The listing builds one solid part. Answer for the finished solid, in the listing's coordinates (mm). A direction names the side the tool comes from. Coordinates: 2 decimals unless noted, no trailing zeros. Order: outer loops, then holes, each group sorted by start corner. A loop starts at its lowest first (then second) coordinate and runs counter-clockwise, first axis right, second up.
```python
from build123d import *

# Parameters (mm, degrees)
SKETCH1_W           = 25.4
SKETCH1_H           = 50.8
SKETCH1_W_2         = 19.05
SKETCH1_H_2         = 44.45
BOSS_EXTRUDE1_DEPTH = 431.8
SKETCH2_R           = 2.54
CUT_EXTRUDE1_DEPTH  = 436.519276267
SKETCH3_R           = 2.54
CUT_EXTRUDE2_DEPTH  = 436.519276267


with BuildPart() as part:
    # Sketch1 → Boss-Extrude1 (new body)
    with BuildSketch(Plane.XY):
        with Locations((12.7, 25.4)):
            Rectangle(SKETCH1_W, SKETCH1_H)
        with Locations((12.7, 25.4)):
            Rectangle(SKETCH1_W_2, SKETCH1_H_2, mode=Mode.SUBTRACT)
    extrude(amount=BOSS_EXTRUDE1_DEPTH)

    # Sketch2 → Cut-Extrude1 (cut, through all)
    with BuildSketch(Plane(origin=(0, 50.8, 0), x_dir=(1, 0, 0), z_dir=(0, 1, 0))):
        with Locations(Location((12.7, -12.7, 0), (0, 0, 270))):
            Circle(SKETCH2_R)
        with Locations(Location((13.029725146, -25.4, 0), (0, 0, 270))):
            Circle(SKETCH2_R)
        with Locations(Location((13.029725146, -38.1, 0), (0, 0, 270))):
            Circle(SKETCH2_R)
        with Locations(Location((13.029725146, -406.4, 0), (0, 0, 270))):
            Circle(SKETCH2_R)
        with Locations(Location((13.029725146, -419.1, 0), (0, 0, 270))):
            Circle(SKETCH2_R)
        with Locations(Location((13.029725146, -393.7, 0), (0, 0, 270))):
            Circle(SKETCH2_R)
        with Locations(Location((13.029725146, -368.3, 0), (0, 0, 270))):
            Circle(SKETCH2_R)
        with Locations(Location((13.029725146, -317.5, 0), (0, 0, 270))):
            Circle(SKETCH2_R)
        with Locations(Location((13.029725146, -266.7, 0), (0, 0, 270))):
            Circle(SKETCH2_R)
        with Locations(Location((13.029725146, -215.9, 0), (0, 0, 270))):
            Circle(SKETCH2_R)
        with Locations(Location((13.029725146, -165.1, 0), (0, 0, 270))):
            Circle(SKETCH2_R)
        with Locations(Location((13.029725146, -114.3, 0), (0, 0, 270))):
            Circle(SKETCH2_R)
        with Locations(Location((13.029725146, -63.5, 0), (0, 0, 270))):
            Circle(SKETCH2_R)
    extrude(amount=-CUT_EXTRUDE1_DEPTH, mode=Mode.SUBTRACT)

    # Sketch3 → Cut-Extrude2 (cut, through all)
    with BuildSketch(Plane(origin=(25.4, 0, 0), x_dir=(0, 0, -1), z_dir=(1, 0, 0))):
        with Locations((-381, 25.4)):
            Circle(SKETCH3_R)
        with Locations((-355.6, 25.4)):
            Circle(SKETCH3_R)
        with Locations((-330.2, 25.4)):
            Circle(SKETCH3_R)
        with Locations((-304.8, 25.4)):
            Circle(SKETCH3_R)
        with Locations((-279.4, 25.4)):
            Circle(SKETCH3_R)
        with Locations((-254, 25.4)):
            Circle(SKETCH3_R)
        with Locations((-228.6, 25.4)):
            Circle(SKETCH3_R)
        with Locations((-203.2, 25.4)):
            Circle(SKETCH3_R)
        with Locations((-177.8, 25.4)):
            Circle(SKETCH3_R)
        with Locations((-152.4, 25.4)):
            Circle(SKETCH3_R)
        with Locations((-127, 25.4)):
            Circle(SKETCH3_R)
        with Locations((-101.6, 25.4)):
            Circle(SKETCH3_R)
        with Locations((-76.2, 25.4)):
            Circle(SKETCH3_R)
        with Locations((-50.8, 25.4)):
            Circle(SKETCH3_R)
    extrude(amount=-CUT_EXTRUDE2_DEPTH, mode=Mode.SUBTRACT)


solid = part.part
```
(1) This flat-tipped pin is pushed along its axis until it touches: pin 1 Ø5 at (x, y) = (7, 11.5) entering from -Z. Where does it stop, or does it pass through?
(2) For faces 5 (the face through (3.175, 25, 213)), 6 (the face through (13, 50.8, 213)), determine the directions among +Z, -Z, +X, -X, +Y, -Y from which every point of the face is accessible in a straight line to the end or side of a thin tool.
(3) Find section B-B (z = 144). Write down the section's boundary in (x, y) (3 decimals).
(4) The mould has two halves that part along Y. Classify faces 1 (the face through (13, 0, 213)), 2 (the face through (13, 47.625, 213)), 3 (the face through (0, 25, 213)), 4 (the face through (22.225, 25, 213)): released by +Y, released by -Y, zero draft, split by the parting line, or undercut.
(5) Find section A-A (y = 39). Write down the section's boundary in (x, z) (3 decimals).
(6) Consider line 1 (Y direction, x = 20.5, z = 46.5) (3 decimals); line 2 (Y direction, x = 23.4, z = 304.8); line 3 (X direction, y = 35, z = 186.5) (3 decimals). Determine where each line is inside the solid, lowest interval first.
Findings below:
1. pin 1: passes through
2. face 5: +Z, -Z
2. face 6: +Z, -Z, +X, -X, +Y
3. outline: (0, 0) - (25.4, 0) - (25.4, 50.8) - (0, 50.8) - close; hole (3.175, 3.175) - (22.225, 3.175) - (22.225, 47.625) - (3.175, 47.625) - close
4. face 1: released by -Y
4. face 2: undercut
4. face 3: zero draft
4. face 4: undercut
5. outline: (0, 0) - (3.175, 0) - (3.175, 431.8) - (0, 431.8) - close; (22.225, 0) - (25.4, 0) - (25.4, 431.8) - (22.225, 431.8) - close
6. line 1: y = 0 to 3.175, 47.625 to 50.8
6. line 2: y = 0 to 22.86, 27.94 to 50.8
6. line 3: x = 0 to 3.175, 22.225 to 25.4
